Verification items for the finished model (mm, model axes). Coordinates: 2 decimals unless noted, no trailing zeros. Write each loop counter-clockwise with the first axis right and the second up, starting at its lowest first coordinate (ties: lowest second). Pieces come first, ordered by that corner, then holes. Notation, with made-up numbers: (-15.5, 82) -> (42.5, 82) arc R17 cw to (42.5, 95) -> close; hole circle Ø1 at (-6.5, -15.75). An arc over 180 degrees is marked (long way). Write item = value, one per line. Start each with the question number.
(1) Mould release check, pull along Z, two halves, no side actions. Record for faces 1 (the face through (-4.88, -0.04, 3.11)), 2 (the face through (9.525, 0, 3)), 3 (the face through (2, 0, 6.35)): released by +Z, released by -Z, zero draft, split by the parting line, or undercut.
(2) Section check A-A (y = 0). Record the cut outline in (x, z) (3 decimals), plus the area to 3 significant figures.
(3) Section check D-D (y = 1.25). Record the cut outline in (x, z) (3 decimals).
(4) Section check B-B (x = 6.35). Record the cut outline in (y, z) (3 decimals), plus the area to 3 significant figures.
(5) Material ranges on probe 1 along Z at (x, y) = (-6.35, 0.5); probe 2 along X at (y, z) = (0.75, 3.5) (3 decimals); probe 3 along X at (y, z) = (-0.5, 2) (3 decimals), recorded low to high. Write a range as [from, to].
(6) Section check C-C (z = 5.5). Record the cut outline in (x, y) (3 decimals), plus the area to 3 significant figures.
```python
from build123d import *

# Parameters (mm, degrees)
SKETCH1_W             = 19.05
SKETCH1_H             = 6.35
BOSS_EXTRUDE1_DEPTH   = 6.35
F_4_CLEARANCE_HOLE1_D = 2.9464
F_4_CLEARANCE_HOLE2_D = 2.9464


with BuildPart() as part:
    # Sketch1 → Boss-Extrude1 (new body)
    with BuildSketch(Plane.XY):
        Rectangle(SKETCH1_W, SKETCH1_H)
    extrude(amount=BOSS_EXTRUDE1_DEPTH)

    # #4 Clearance Hole1 (through all)
    with Locations(Plane(origin=(0, 3.175, 0), x_dir=(1, 0, 0), z_dir=(0, 1, 0))):
        with Locations((-6.35, -3.175), (6.35, -3.175)):
            Hole(F_4_CLEARANCE_HOLE1_D / 2)

    # #4 Clearance Hole2 (through all)
    with Locations(Plane.XY.offset(6.35)):
        with Locations((0, 0)):
            Hole(F_4_CLEARANCE_HOLE2_D / 2)


solid = part.part
```
Response:
q1.face_1 = undercut
q1.face_2 = zero draft
q1.face_3 = released by +Z
q2.outline = (-9.525, 0) -> (-1.473, 0) -> (-1.473, 6.35) -> (-9.525, 6.35) -> close; (1.473, 0) -> (9.525, 0) -> (9.525, 6.35) -> (1.473, 6.35) -> close; hole circle Ø2.946 at (-6.35, 3.175); hole circle Ø2.946 at (6.35, 3.175)
q2.area = 88.6 mm2
q3.outline = (-9.525, 0) -> (-0.78, 0) -> (-0.78, 6.35) -> (-9.525, 6.35) -> close; (0.78, 0) -> (9.525, 0) -> (9.525, 6.35) -> (0.78, 6.35) -> close; hole circle Ø2.946 at (-6.35, 3.175); hole circle Ø2.946 at (6.35, 3.175)
q4.outline = (-3.175, 0) -> (3.175, 0) -> (3.175, 1.702) -> (-3.175, 1.702) -> close; (-3.175, 4.648) -> (3.175, 4.648) -> (3.175, 6.35) -> (-3.175, 6.35) -> close
q4.area = 21.6 mm2
q5.probe_1 = [0, 1.7], [4.65, 6.35]
q5.probe_2 = [-9.525, -7.787], [-4.913, -1.268], [1.268, 4.913], [7.787, 9.525]
q5.probe_3 = [-9.525, -7.239], [-5.461, -1.386], [1.386, 5.461], [7.239, 9.525]
q6.outline = (-9.525, -3.175) -> (9.525, -3.175) -> (9.525, 3.175) -> (-9.525, 3.175) -> close; hole circle Ø2.946 at (0, 0)
q6.area = 114 mm2
